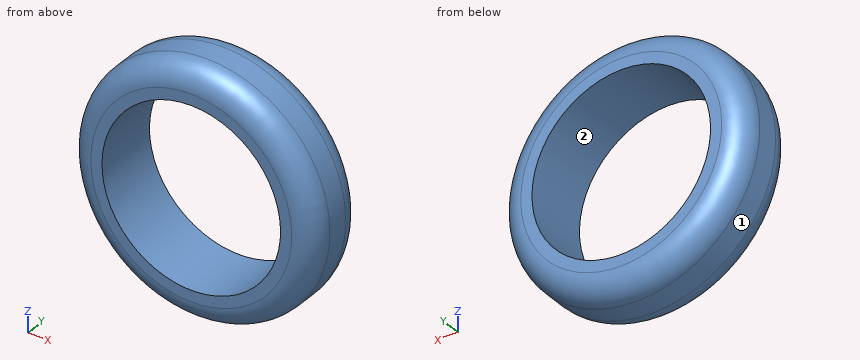
```python
from build123d import *

# Parameters (mm, degrees)
CROQUIS1_R              = 5.5
SALIENTE_EXTRUIR1_DEPTH = 3
CROQUIS2_R              = 4
CORTAR_EXTRUIR1_DEPTH   = 5
REDONDEO1_R             = 1
REDONDEO2_R             = 1


with BuildPart() as part:
    # Croquis1 → Saliente-Extruir1 (new body)
    with BuildSketch(Plane(origin=(0, 0, 0), x_dir=(1, 0, 0), z_dir=(0, 1, 0))):
        with Locations(Location((0, 0, 0), (0, 0, 270))):
            Circle(CROQUIS1_R)
    extrude(amount=SALIENTE_EXTRUIR1_DEPTH)

    # Croquis2 → Cortar-Extruir1 (cut)
    with BuildSketch(Plane(origin=(0, 3, 0), x_dir=(1, 0, 0), z_dir=(0, 1, 0))):
        with Locations(Location((0, 0, 0), (0, 0, 270))):
            Circle(CROQUIS2_R)
    extrude(amount=-CORTAR_EXTRUIR1_DEPTH, mode=Mode.SUBTRACT)

    # Redondeo1
    redondeo1_edges = [part.edges().sort_by_distance(p)[0] for p in [
        (0, 3, -5.5),
    ]]
    fillet(redondeo1_edges, radius=REDONDEO1_R)

    # Redondeo2
    redondeo2_edges = [part.edges().sort_by_distance(p)[0] for p in [
        (0, 0, -5.5),
    ]]
    fillet(redondeo2_edges, radius=REDONDEO2_R)


solid = part.part
```
Read the model definition and answer for the solid it produces. Units are mm, in the model's axes. Face numbers are marked on the shaded views. Give positions to 0.01 mm unless a question says otherwise; leave off trailing zeros. Loops run counter-clockwise (first coordinate to the right, second up) from the corner with the lowest first, then second, coordinate; pieces in that order, holes last.
Item 1: The part is cut by section C-C (y = 1.15). Write down the section's boundary in (x, z), and give its area (3 significant figures).
Item 2: The part is cut by section A-A (z = 0). Write down the section's boundary in (x, y).
Item 3: The mould has two halves that part along Z. Classify the marked faces 1 and 2: released by +Z, released by -Z, zero draft, split by the parting line, or undercut.
Item 4: The part is cut by section D-D (y = 0.45). Write down the section's boundary in (x, z).
Item 5: The part is cut by section B-B (x = 0). Write down the section's boundary in (y, z).
Item 6: Find the intervals of material crossed by line 1 along X through (y, z) = (1.6, 0); line 2 along X through (y, z) = (2.25, -0.5); line 3 along Z through (x, y) = (-3.5, 1.2), in increasing order.
Taken from the geometry:
1. outline: circle Ø11 at (0, 0); hole circle Ø8 at (0, 0)
1. area: 44.8 mm2
2. outline: (-5.5, 1) arc R1 ccw to (-4.5, 0) - (-4, 0) - (-4, 3) - (-4.5, 3) arc R1 ccw to (-5.5, 2) - close; (4, 0) - (4.5, 0) arc R1 ccw to (5.5, 1) - (5.5, 2) arc R1 ccw to (4.5, 3) - (4, 3) - close
3. face 1: split by the parting line
3. face 2: undercut
4. outline: circle Ø10.67 at (0, 0); hole circle Ø8 at (0, 0)
5. outline: (0, -4.5) arc R1 ccw to (1, -5.5) - (2, -5.5) arc R1 ccw to (3, -4.5) - (3, -4) - (0, -4) - close; (0, 4) - (3, 4) - (3, 4.5) arc R1 ccw to (2, 5.5) - (1, 5.5) arc R1 ccw to (0, 4.5) - close
6. line 1: x = -5.5 to -4, 4 to 5.5
6. line 2: x = -5.45 to -3.97, 3.97 to 5.45
6. line 3: z = -4.24 to -1.94, 1.94 to 4.24
